Can you work these out from the model? Positions are in its coordinate system, mm. Face numbers are marked on the shaded views. Give positions to 0.01 mm unless a question says otherwise; leave off trailing zeros. Order: outer loops, then holes, each group sorted by start corner. A loop starts at its lowest first (then second) coordinate and runs counter-clockwise, first axis right, second up. Notation, with made-up numbers: (-13, -16.5) - (18, -16.5) arc R35 cw to (18, 20.5) - close; hole circle Ø9 at (-33.5, 15). An arc over 180 degrees is marked (long way). Answer as CSV lines item,"result".
```python
from build123d import *

# Parameters (mm, degrees)
SKETCH1_W            = 33
SKETCH1_H            = 39.4
BOSS_EXTRUDE1_DEPTH  = 9.525
M3_CLEARANCE_HOLE1_D = 3.2
M4_CLEARANCE_HOLE1_D = 4.3
FILLET1_R            = 2


with BuildPart() as part:
    # Sketch1 → Boss-Extrude1 (new body)
    with BuildSketch(Plane.XY):
        Rectangle(SKETCH1_W, SKETCH1_H)
    extrude(amount=BOSS_EXTRUDE1_DEPTH)

    # M3 Clearance Hole1 (through all)
    with Locations(Plane.XY.offset(9.525)):
        with Locations((-10, 0), (0, 0), (10, 0)):
            Hole(M3_CLEARANCE_HOLE1_D / 2)

    # M4 Clearance Hole1 (through all)
    with Locations(Plane.XY.offset(9.525)):
        with Locations((-13, 13), (-13, -13), (13, -13), (13, 13)):
            Hole(M4_CLEARANCE_HOLE1_D / 2)

    # Fillet1
    fillet1_edges = [part.edges().sort_by_distance(p)[0] for p in [
        (-16.5, 19.7, 4.7625),
        (16.5, 19.7, 4.7625),
        (16.5, -19.7, 4.7625),
        (-16.5, -19.7, 4.7625),
    ]]
    fillet(fillet1_edges, radius=FILLET1_R)


solid = part.part
```
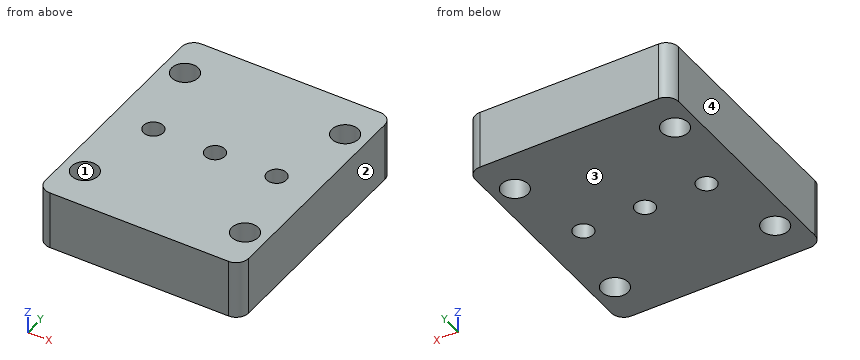
1) If we mould it in two halves opening along X, with no side actions, what happens to the marked faces 1, 2, 3 and 4? For each: +X half, -X half, draft (parallel to the pull), parting line (faces both ways), or undercut.
Answer block:
face 1,"undercut"
face 2,"+X half"
face 3,"draft"
face 4,"-X half"
2) I want a section at B-B on y = 13. Write out the boundary of the cut face in (x, z) (3 decimals).
Answer block:
outline,"(-16.5, 0) - (-15.15, 0) - (-15.15, 9.525) - (-16.5, 9.525) - close; (-10.85, 0) - (10.85, 0) - (10.85, 9.525) - (-10.85, 9.525) - close; (15.15, 0) - (16.5, 0) - (16.5, 9.525) - (15.15, 9.525) - close"
3) I need wall thicknesses on line 1 along Y through (x, z) = (-13, 5); line 2 along Y through (x, z) = (0, 7.5); line 3 along Y through (x, z) = (12, 1.75). Which ranges of each line are inside material? Lowest first, please. Write a range as [from, to].
Answer block:
line 1,"[-19.7, -15.15], [-10.85, 10.85], [15.15, 19.7]"
line 2,"[-19.7, -1.6], [1.6, 19.7]"
line 3,"[-19.7, -14.9], [-11.1, 11.1], [14.9, 19.7]"
4) I want a section at C-C on z = 8.25. Write out the boundary of the cut face in (x, y).
Answer block:
outline,"(-16.5, -17.7) arc R2 ccw to (-14.5, -19.7) - (14.5, -19.7) arc R2 ccw to (16.5, -17.7) - (16.5, 17.7) arc R2 ccw to (14.5, 19.7) - (-14.5, 19.7) arc R2 ccw to (-16.5, 17.7) - close; hole circle Ø4.3 at (-13, -13); hole circle Ø4.3 at (-13, 13); hole circle Ø3.2 at (-10, 0); hole circle Ø3.2 at (0, 0); hole circle Ø3.2 at (10, 0); hole circle Ø4.3 at (13, -13); hole circle Ø4.3 at (13, 13)"
5) I want a section at A-A on x = 10. Write out the boundary of the cut face in (y, z) (3 decimals), plus the area to 3 significant figures.
Answer block:
outline,"(-19.7, 0) - (-1.6, 0) - (-1.6, 9.525) - (-19.7, 9.525) - close; (1.6, 0) - (19.7, 0) - (19.7, 9.525) - (1.6, 9.525) - close"
area,"345 mm2"
6) I want a section at D-D on x = -13. Write out the boundary of the cut face in (y, z) (3 decimals), plus the area to 3 significant figures.
Answer block:
outline,"(-19.7, 0) - (-15.15, 0) - (-15.15, 9.525) - (-19.7, 9.525) - close; (-10.85, 0) - (10.85, 0) - (10.85, 9.525) - (-10.85, 9.525) - close; (15.15, 0) - (19.7, 0) - (19.7, 9.525) - (15.15, 9.525) - close"
area,"293 mm2"
